Geometry check sheet. Reference: drawing and pictorial views, mm from the part's lowest x, y, z. Coordinates: 2 decimals unless noted, no trailing zeros. Order: outer loops, then holes, each group sorted by start corner. A loop starts at its lowest first (then second) coordinate and runs counter-clockwise, first axis right, second up. Notation, with made-up numbers: M 80,42.25 L 127,42.25 A23 ccw 127,60.25 Z; hole C 3,79.5 d6. An arc over 180 degrees is marked long. Return JSON: item names as keys, results as strings.
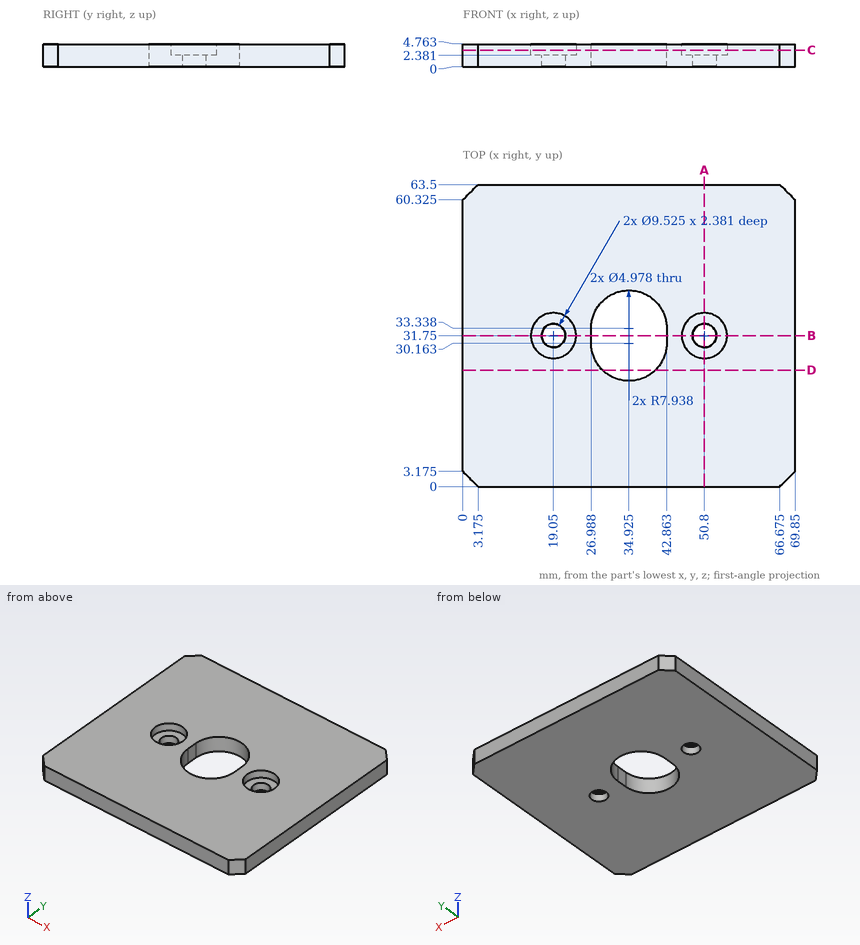
Q1. Cross-section at D-D, the plane y = 24.5. Record the boundary of the cut face in (x, z).
Values:
{"outline": "M 0,0 L 29.36,0 L 29.36,4.76 L 0,4.76 Z; M 40.49,0 L 69.85,0 L 69.85,4.76 L 40.49,4.76 Z"}
Q2. Material ranges on line 1 along Y through (x, z) = (15, 2.5) (1 decimal); line 2 along Y through (x, z) = (50.8, 0.55), recorded low to high.
Values:
{"line 1": "0 to 29.2, 34.3 to 63.5", "line 2": "0 to 29.26, 34.24 to 63.5"}
Q3. Cross-section at B-B, the plane y = 31.75. Record the boundary of the cut face in (x, z), and give its area (3 significant figures).
Values:
{"outline": "M 0,0 L 16.56,0 L 16.56,2.38 L 14.29,2.38 L 14.29,4.76 L 0,4.76 Z; M 21.54,0 L 26.99,0 L 26.99,4.76 L 23.81,4.76 L 23.81,2.38 L 21.54,2.38 Z; M 42.86,0 L 48.31,0 L 48.31,2.38 L 46.04,2.38 L 46.04,4.76 L 42.86,4.76 Z; M 53.29,0 L 69.85,0 L 69.85,4.76 L 55.56,4.76 L 55.56,2.38 L 53.29,2.38 Z", "area": "188 mm^2"}
Q4. Cross-section at A-A, the plane x = 50.8. Record the boundary of the cut face in (y, z), and give its area (3 significant figures).
Values:
{"outline": "M 0,0 L 29.26,0 L 29.26,2.38 L 26.99,2.38 L 26.99,4.76 L 0,4.76 Z; M 34.24,0 L 63.5,0 L 63.5,4.76 L 36.51,4.76 L 36.51,2.38 L 34.24,2.38 Z", "area": "268 mm^2"}
Q5. Go/stop test with flat-tipped pins: pin 1 (15 mm diameter, centred on x = 19.05, y = 31.75, fed in from -Z); pin 2 (8.5 mm diameter, centred on x = 50.8, y = 31.75, fed in from +Z). Record where each tip stops, or that it passes through.
Values:
{"pin 1": "z = 0", "pin 2": "z = 2.38"}
Q6. Cross-section at C-C, the plane z = 3.45. State how many separate pieces and enclosed holes the cut face has, and give its area (3 significant figures).
Values:
{"separate pieces": "1", "enclosed holes": "3", "area": "4,020 mm^2"}
